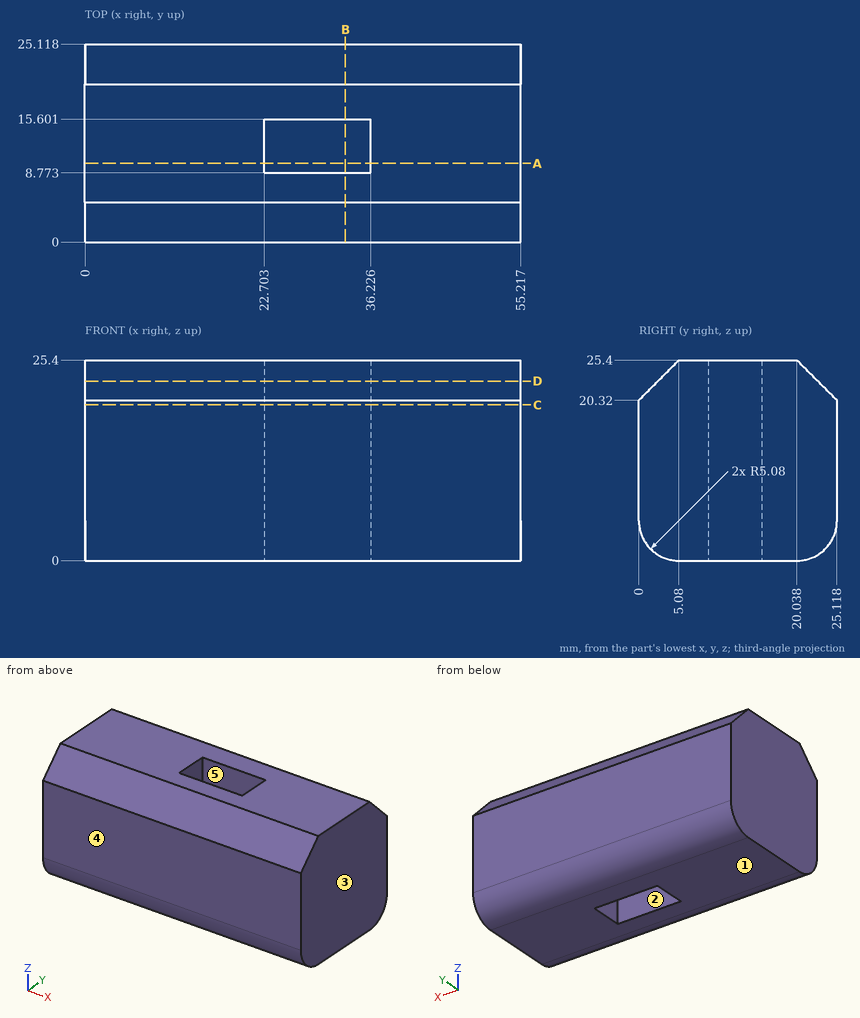
Here's the drawing with two shaded views (mm, measured from the low corner). I have some questions. A direction names the side the tool comes from. Coordinates: 2 decimals unless noted, no trailing zeros. Write each loop counter-clockwise with the first axis right and the second up, starting at its lowest first coordinate (ties: lowest second). Pieces come first, ordered by that corner, then holes. Notation, with made-up numbers: (35.25, -1) -> (66.25, -1) arc R22 cw to (66.25, 8) -> close; hole circle Ø9 at (40, 1.5). An arc over 180 degrees is marked (long way). Use a Markdown table: item, result. Add a question column.
(1) We'd pull the mould along X, two halves only. Please class the marked faces 1, 2 and 3: +X half, -X half, draft (parallel to the pull), parting line (faces both ways), or undercut.
(2) If we section it at B-B, the plane x = 33: Write out the boundary of the cut face in (y, z).
(3) I'm going to push a flat-ended pin straight in: P1, Ø1, axis at x = 24.5, y = 3, coming from the -Z side. Where does the tip first touch, or does it pass through?
(4) For the marked faces 4 and 5, which set-ups out of +Z, -Z, +X, -X, +Y, -Y let a thin tool reach every point of the face, with its end or its side?
(5) Please list where these lines run through material, in increasing order: line 1 (X direction, y = 9, z = 6.75) (1 decimal); line 2 (Y direction, x = 27, z = 10); line 3 (Y direction, x = 25.5, z = 23.75).
(6) If we section it at A-A, the plane y = 10: Write out the boundary of the cut face in (x, z) (1 decimal), and give its area (3 significant figures).
(7) If we section it at D-D, the plane z = 22.75: Write out the boundary of the cut face in (x, y) (1 decimal), and give its area (3 significant figures).
(8) If we section it at C-C, the plane z = 19.75: Write out the boundary of the cut face in (x, y) (1 decimal).
Outcome:
| question | item | result |
|---|---|---|
| 1 | face 1 | draft |
| 1 | face 2 | undercut |
| 1 | face 3 | +X half |
| 2 | outline | (0, 5.08) arc R5.08 ccw to (5.08, 0) -> (8.77, 0) -> (8.77, 25.4) -> (5.08, 25.4) -> (0, 20.32) -> close; (15.6, 0) -> (20.04, 0) arc R5.08 ccw to (25.12, 5.08) -> (25.12, 20.32) -> (20.04, 25.4) -> (15.6, 25.4) -> close |
| 3 | P1 | stops at z = 0.25 |
| 4 | face 4 | +Z, -Z, +X, -X, -Y |
| 4 | face 5 | +Z, -Z |
| 5 | line 1 | x = 0 to 22.7, 36.2 to 55.2 |
| 5 | line 2 | y = 0 to 8.77, 15.6 to 25.12 |
| 5 | line 3 | y = 3.43 to 8.77, 15.6 to 21.69 |
| 6 | outline | (0, 0) -> (22.7, 0) -> (22.7, 25.4) -> (0, 25.4) -> close; (36.2, 0) -> (55.2, 0) -> (55.2, 25.4) -> (36.2, 25.4) -> close |
| 6 | area | 1,060 mm^2 |
| 7 | outline | (0, 2.4) -> (55.2, 2.4) -> (55.2, 22.7) -> (0, 22.7) -> close; hole (22.7, 8.8) -> (36.2, 8.8) -> (36.2, 15.6) -> (22.7, 15.6) -> close |
| 7 | area | 1,030 mm^2 |
| 8 | outline | (0, 0) -> (55.2, 0) -> (55.2, 25.1) -> (0, 25.1) -> close; hole (22.7, 8.8) -> (36.2, 8.8) -> (36.2, 15.6) -> (22.7, 15.6) -> close |
